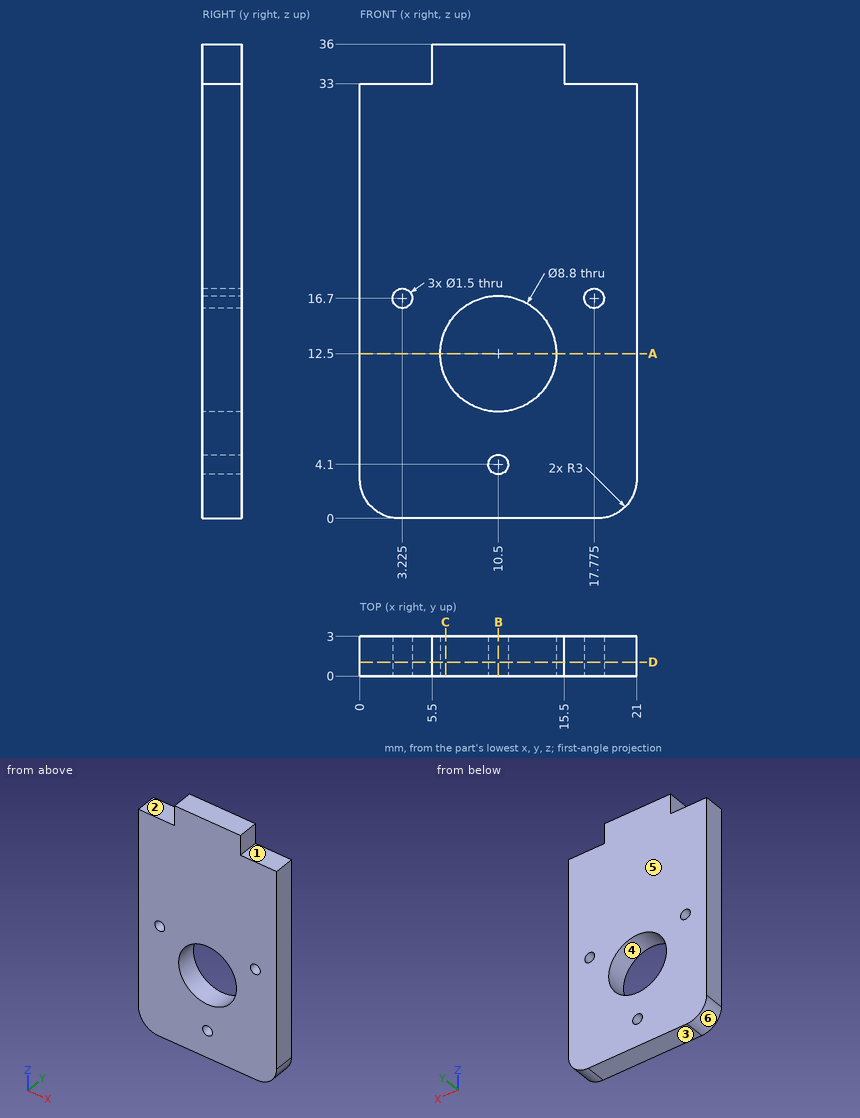
Design review of the part shown in the three views and the two pictorial views. Dimensions are in mm from the part's minimum x, y and z. A direction names the side the tool comes from. Round coordinates to 2 decimals unless told otherwise and drop trailing zeros. Write each loop counter-clockwise with the first axis right and the second up, starting at its lowest first coordinate (ties: lowest second). Pieces come first, ordered by that corner, then holes. Notation, with made-up numbers: (72, 22) - (92, 22) arc R7 cw to (92, 26) - close; hole circle Ø7 at (45, 26.5). An arc over 180 degrees is marked (long way). Return JSON: item names as keys, results as strings. Group by question number.
Item 1: We need section B-B on x = 10.5. Write out the cut boundary in (y, z).
Item 2: The part is to be moulded in two halves that separate along X. For the marked faces 4, 5 and 6, say which applies: pulls with the +X half, pulls with the -X half, needs draft (parallel to the pull), parting line crosses it, or undercut.
Item 3: Machinability: for the marked faces 1, 2 and 3, which of the approach directions +Z, -Z, +X, -X, +Y, -Y give a long, thin tool a straight path to every point of the face, cutting with its end or side? Answer none if there is none.
Item 4: We need section A-A on z = 12.5. Write out the cut boundary in (x, y), and give its area (3 significant figures).
Item 5: For probe 1 along Z at (x, y) = (10.75, 0.3); probe 2 along Z at (x, y) = (17.75, 2); probe 3 along Z at (x, y) = (11, 2.45), list the stretches that pass through material, from the lowest coordinate up. Write a range as [from, to].
Item 6: Insertion check: P1, Ø2.5, axis at x = 10.5, z = 4.1, coming from the -Y side; P2, Ø1.5, axis at x = 17.5, y = 2, coming from the +Z side; P3, Ø1.5, axis at y = 1, z = 34, coming from the -X side; P4, Ø7, axis at x = 10.5, z = 12.5, coming from the +Y side. Each pin has a flat end and moves straight along its axis. Give the tip position at first contact, or say it passes through.
Item 7: We need section C-C on x = 6.5. Write out the cut boundary in (y, z).
Item 8: We need section D-D on y = 1.05. Give the number of separate pieces and of enclosed holes in the cut face, and give its area (3 significant figures).
Model answer:
{
 "1": {"outline": "(0, 0) - (3, 0) - (3, 3.35) - (0, 3.35) - close; (0, 4.85) - (3, 4.85) - (3, 8.1) - (0, 8.1) - close; (0, 16.9) - (3, 16.9) - (3, 36) - (0, 36) - close"},
 "2": {"face 4": "undercut", "face 5": "needs draft", "face 6": "pulls with the -X half"},
 "3": {"face 1": "+Z, +X, +Y, -Y", "face 2": "+Z, -X, +Y, -Y", "face 3": "-Z, +X, -X, +Y, -Y"},
 "4": {"outline": "(0, 0) - (6.1, 0) - (6.1, 3) - (0, 3) - close; (14.9, 0) - (21, 0) - (21, 3) - (14.9, 3) - close", "area": "36.6 mm²"},
 "5": {"probe 1": "z = [0, 3.39], [4.81, 8.11], [16.89, 36]", "probe 2": "z = [0, 15.95], [17.45, 33]", "probe 3": "z = [0, 3.54], [4.66, 8.13], [16.87, 36]"},
 "6": {"P1": "stops at y = 0", "P2": "stops at z = 33", "P3": "stops at x = 5.5", "P4": "passes through"},
 "7": {"outline": "(0, 0) - (3, 0) - (3, 10.67) - (0, 10.67) - close; (0, 14.33) - (3, 14.33) - (3, 36) - (0, 36) - close"},
 "8": {"separate pieces": "1", "enclosed holes": "4", "area": "653 mm²"}
}
